```python
from build123d import *

# Parameters (mm, degrees)
F1_DEPTH    = 48
F0_W        = 42
F0_H        = 14
F2_DEPTH    = 10
F3_T1_DEPTH = 24
F4_T1_DEPTH = 24
F5_R        = 6
F6_DEPTH    = 3
F5_W        = 28
F5_H        = 5
F7_DEPTH    = 3
F8_R        = 6
F9_R        = 6
F10_W       = 28
F10_H       = 5
F11_DEPTH   = 5


# Not quite as in the source:
# - a fillet or chamfer that OpenCascade refuses, or shapes differently, is made with other operations: its cross-section is extruded or revolved along the edge and cut away or added


with BuildPart() as f1:
    # F0 (on Top) → F1 (new body)
    with BuildSketch(Plane.XY):
        Polygon((31, 0), (31, 24), (21, 24), (21, 10), (-21, 10), (-21, 24), (-31, 24), (-31, 0), align=None)
    extrude(amount=F1_DEPTH)

    # F0 (on Top) → F2 (join)
    with BuildSketch(Plane.XY):
        Polygon((-46, -24), (46, -24), (46, 24), (31, 24), (31, 0), (-31, 0), (-31, 24), (-46, 24), align=None)
        Polygon((31, 0), (31, 24), (21, 24), (21, 10), (-21, 10), (-21, 24), (-31, 24), (-31, 0), align=None)
        with Locations((0, 17)):
            Rectangle(F0_W, F0_H)
    extrude(amount=F2_DEPTH)

    # F3: fillet of radius 25 on 1 edges, made by hand

    # F3_s2 → F3_t1 (join)
    with BuildSketch(Plane.XZ.offset(-24)):
        with BuildLine():
            ThreePointArc((46, 10), (35.0834993366, 19.2198145372), (31, 32.9128784748))
            Line((31, 32.9128784748), (31, 10))
            Line((31, 10), (46, 10))
        make_face()
    extrude(amount=F3_T1_DEPTH)

    # F4: fillet of radius 25 on 1 edges, made by hand

    # F4_s2 → F4_t1 (join)
    with BuildSketch(Plane.XZ.offset(-24)):
        with BuildLine():
            ThreePointArc((-31, 32.9128784748), (-35.0834993366, 19.2198145372), (-46, 10))
            Line((-46, 10), (-31, 10))
            Line((-31, 10), (-31, 32.9128784748))
        make_face()
    extrude(amount=F4_T1_DEPTH)

    # F5 (on face) → F6 (join)
    with BuildSketch(Plane.XZ):
        with BuildLine():
            Line((14, 15), (14, 29))
            ThreePointArc((14, 29), (0, 43), (-14, 29))
            Line((-14, 29), (-14, 15))
            Line((-14, 15), (14, 15))
        make_face()
        with Locations((0, 29)):
            Circle(F5_R, mode=Mode.SUBTRACT)
    extrude(amount=F6_DEPTH)

    # F5 (on face) → F7 (join)
    with BuildSketch(Plane.XZ):
        with BuildLine():
            Line((14, 15), (14, 29))
            ThreePointArc((14, 29), (0, 43), (-14, 29))
            Line((-14, 29), (-14, 15))
            Line((-14, 15), (14, 15))
        make_face()
        with Locations((0, 29)):
            Circle(F5_R, mode=Mode.SUBTRACT)
        with Locations((0, 12.5)):
            Rectangle(F5_W, F5_H)
    extrude(amount=F7_DEPTH)

    # F8
    f8_edges = [f1.edges().sort_by_distance(p)[0] for p in [
        (46, -24, 5),
    ]]
    fillet(f8_edges, radius=F8_R)

    # F9
    f9_edges = [f1.edges().sort_by_distance(p)[0] for p in [
        (-46, -24, 5),
    ]]
    fillet(f9_edges, radius=F9_R)

    # F10 (on face) → F11 (join)
    with BuildSketch(Plane.XZ):
        with Locations((0, 12.5)):
            Rectangle(F10_W, F10_H)
    extrude(amount=F11_DEPTH)


solid = f1.part
```
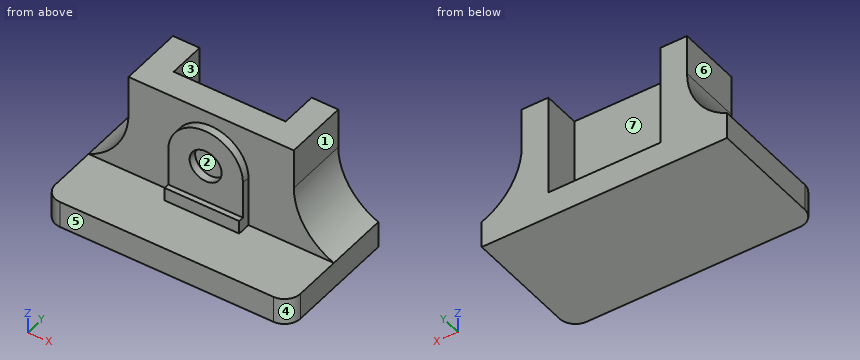
Geometry check sheet. Reference: the model listing, model coordinates, mm. Face numbers are marked on the shaded views. A direction names the side the tool comes from. Give positions to 0.01 mm unless a question says otherwise; leave off trailing zeros. Order: outer loops, then holes, each group sorted by start corner. A loop starts at its lowest first (then second) coordinate and runs counter-clockwise, first axis right, second up.
1. Release check for a two-part mould opening along X. For the marked faces 4, 5, 6 and 7 record: pulls with the +X half, pulls with the -X half, needs draft (parallel to the pull), parting line crosses it, or undercut.
2. Section check A-A, the plane x = 0. Enter the section's corners in (y, z).
3. Thickness scan on L1, parallel to Z at x = 0, y = -1; L2, parallel to Y at x = 22.5, z = 15.5; L3, parallel to Z at x = -22.5, y = -16.5. Record the ranges inside material, lowest first.
4. Section check C-C, the plane z = 38.5. Enter the section's corners in (x, y).
5. Section check D-D, the plane x = 30. Enter the section's corners in (y, z), and give its area (3 significant figures).
6. Access from +Z, -Z, +X, -X, +Y, -Y to the whole of each face (thin tool, end or side, straight path). Record for the marked faces 1, 2 and 3.
7. Section check B-B, the plane y = 14. Enter the section's corners in (x, z), and give its area (3 significant figures).
8. Gauge pin test, flat ends, axial feed: pin 1 Ø11 at (y, z) = (18.5, 36.5) entering from -X; pin 2 Ø11 at (x, y) = (7.5, 14) entering from +Z; pin 3 Ø4 at (y, z) = (14, 19.5) entering from +X; pin 4 Ø7.5 at (y, z) = (11.5, 42) entering from +X. Record the tip position at first contact, or that the pin passes through.
Values follow:
1. face 4: pulls with the +X half
1. face 5: needs draft
1. face 6: pulls with the -X half
1. face 7: undercut
2. outline: (-24, 0) - (24, 0) - (24, 10) - (10, 10) - (10, 48) - (0, 48) - (0, 43) - (-3, 43) - (-3, 35) - (0, 35) - (0, 23) - (-3, 23) - (-3, 15) - (-5, 15) - (-5, 10) - (-24, 10) - close
3. L1: z = 0 to 23, 35 to 43
3. L2: y = 0 to 24
3. L3: z = 0 to 10
4. outline: (-31, 0) - (-10.28, 0) - (-10.28, -3) - (10.28, -3) - (10.28, 0) - (31, 0) - (31, 24) - (21, 24) - (21, 10) - (-21, 10) - (-21, 24) - (-31, 24) - close
5. outline: (-24, 0) - (24, 0) - (24, 48) - (0, 48) - (0, 10) - (-24, 10) - close
5. area: 1,390 mm2
6. face 1: +Z, +X, +Y, -Y
6. face 2: -Y
6. face 3: +Z, +Y
7. outline: (-46, 0) - (46, 0) - (46, 10) arc R25 cw to (31, 32.91) - (31, 48) - (21, 48) - (21, 10) - (-21, 10) - (-21, 48) - (-31, 48) - (-31, 32.91) arc R25 cw to (-46, 10) - close
7. area: 1,870 mm2
8. pin 1: stops at x = -31.07
8. pin 2: stops at z = 48
8. pin 3: stops at x = 36.32
8. pin 4: stops at x = 31
